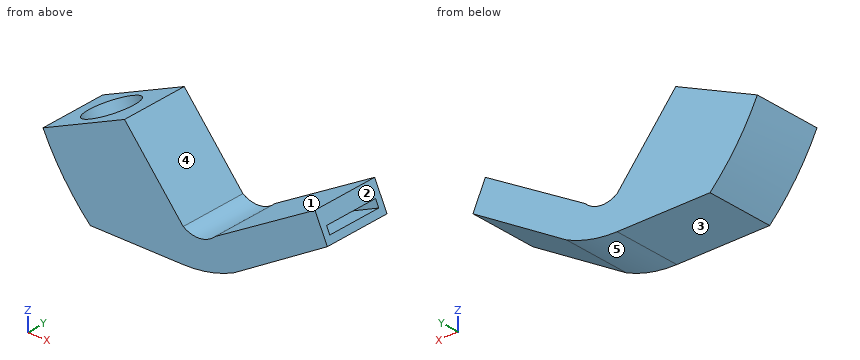
from build123d import *

# Parameters (mm, degrees)
F1_DEPTH = 7.62
F2_DEPTH = 7.62
F3_R     = 2.7444013429
F4_DEPTH = 6.35
F5_W     = 6.2532699667
F5_H     = 0.86275296
F6_DEPTH = 7.62


with BuildPart() as f1:
    # F0 (on Front) → F1 (new body)
    with BuildSketch(Plane.XZ):
        with BuildLine():
            Line((-10.3579089046, 0), (0, 0))
            Line((0, 0), (0, 3.645401448))
            Line((0, 3.645401448), (-6.5403589979, 11.5425735712))
            Line((-6.5403589979, 11.5425735712), (-15.6276854686, 7.4571091682))
            ThreePointArc((-15.6276854686, 7.4571091682), (-13.3121430449, 3.5028798243), (-10.3579089046, 0))
        make_face()
    extrude(amount=F1_DEPTH)

    # F0 (on Front) → F2 (join)
    with BuildSketch(Plane.XZ):
        with BuildLine():
            Line((0, 3.645401448), (0, 0))
            ThreePointArc((0, 0), (2.8721308182, 0.311594991), (5.6106159464, 1.2318808585))
            Line((5.6106159464, 1.2318808585), (16.058837386, 7.5155025299))
            Line((16.058837386, 7.5155025299), (14.6878519678, 10.5192856507))
            Line((14.6878519678, 10.5192856507), (3.5806233063, 3.9957128465))
            ThreePointArc((3.5806233063, 3.9957128465), (1.853653217, 3.1731266591), (0, 3.645401448))
        make_face()
    extrude(amount=F2_DEPTH)

    # F3 (on face) → F4 (cut)
    with BuildSketch(Plane(origin=(-5.4164543998, 0, 12.0478566424), x_dir=(0.9120653953, 0, 0.4100447715), z_dir=(-0.4100447715, 0, 0.9120653953))):
        with Locations((-6.5201530233, -3.7630312145)):
            Circle(F3_R)
    extrude(amount=-F4_DEPTH, mode=Mode.SUBTRACT)

    # F5 (on face) → F6 (cut)
    with BuildSketch(Plane(origin=(16.1290707313, 0, 7.3616236234), x_dir=(0, 1, 0), z_dir=(0.9097231122, 0, 0.4152154371))):
        with Locations((-3.7998675834, 1.3887053062)):
            Rectangle(F5_W, F5_H)
    extrude(amount=-F6_DEPTH, mode=Mode.SUBTRACT)


solid = f1.part
Can you work these out from the model? Positions are in its coordinate system, mm. Face numbers are marked on the shaded views. A direction names the side the tool comes from. Give positions to 0.01 mm unless a question says otherwise; leave off trailing zeros. Order: outer loops, then holes, each group sorted by start corner. A loop starts at its lowest first (then second) coordinate and runs counter-clockwise, first axis right, second up. Notation, with made-up numbers: (82, 32.5) - (100, 32.5) arc R25 ccw to (100, 49.5) - close; hole circle Ø11 at (-31, -29.5). An arc over 180 degrees is marked (long way). Write each question's results on one line, items separated by ' | '.
1) On a 3-axis mill with a long thin cutter (end or side, diameter ignored), from which of +Z, -Z, +X, -X, +Y, -Y can I reach the whole of each face in a straight line? I mean the marked faces 4 and 5. Say none if no direction works.
Final values:
face 4: +Z, +Y, -Y | face 5: -Z, +X, +Y, -Y
2) Suppose I cut it at A-A, the plane z = 6.75. Give the number of separate pieces and of enclosed holes in the cut face, then the cut area to 3 significant figures.
Final values:
separate pieces: 2 | enclosed holes: 2 | area: 108 mm^2
3) I'm going to push flat-ended pins straight in: pin 1 Ø3 at (y, z) = (-6.5, 5) entering from -X; pin 2 Ø1 at (y, z) = (-5.5, 3.5) entering from -X; pin 3 Ø2 at (y, z) = (-2.5, 9.5) entering from +X. Where does each tip first touch, or does it pass through?
Final values:
pin 1: stops at x = -15.15 | pin 2: stops at x = -13.66 | pin 3: stops at x = 15.37
4) Suppose I cut it at B-B, the plane y = -1.5. Write out the boundary of the cut face in (x, z), then the cut area to 3 significant figures.
Final values:
outline: (-15.63, 7.46) arc R26.85 ccw to (-10.36, 0) - (0, 0) arc R13.39 ccw to (5.61, 1.23) - (16.06, 7.52) - (15.73, 8.23) - (8.8, 5.07) - (8.44, 5.85) - (15.37, 9.02) - (14.69, 10.52) - (3.58, 4) arc R2.81 cw to (0, 3.65) - (-6.54, 11.54) - (-9.95, 10.01) - (-7.34, 4.22) - (-10.18, 2.95) - (-12.78, 8.74) - close | area: 150 mm^2
5) Please list where these lines run through material, in increasing order: line 1 along X through (y, z) = (-1.75, 4); line 2 along X through (y, z) = (-1.75, 7); line 3 along X through (y, z) = (-3.75, 6.25). Write a range as [from, to].
Final values:
line 1: x = [-13.66, -10.99], [-7.83, -0.29], [3.59, 10.21] | line 2: x = [-15.4, -12.34], [-8.25, -2.78], [8.7, 10.95], [13.03, 15.2] | line 3: x = [-15.02, -12.97], [-6.95, -2.16], [7.42, 9.31], [11.39, 13.95]
6) Suppose I cut it at C-C, the plane x = 10. Write out the boundary of the cut face in (y, z).
Final values:
outline: (-7.62, 3.87) - (0, 3.87) - (0, 7.77) - (-7.62, 7.77) - close; hole (-6.93, 5.62) - (-0.67, 5.62) - (-0.67, 6.56) - (-6.93, 6.56) - close
7) Suppose I cut it at D-D, the plane x = 13.5. Write out the boundary of the cut face in (y, z).
Final values:
outline: (-7.62, 5.98) - (0, 5.98) - (0, 9.82) - (-7.62, 9.82) - close; hole (-6.93, 7.21) - (-0.67, 7.21) - (-0.67, 8.16) - (-6.93, 8.16) - close
8) If we mould it in two halves opening along X, with no side actions, what happens to the marked faces 1, 2 and 3? For each: pulls with the +X half, pulls with the -X half, needs draft (parallel to the pull), parting line crosses it, or undercut.
Final values:
face 1: undercut | face 2: pulls with the +X half | face 3: needs draft
